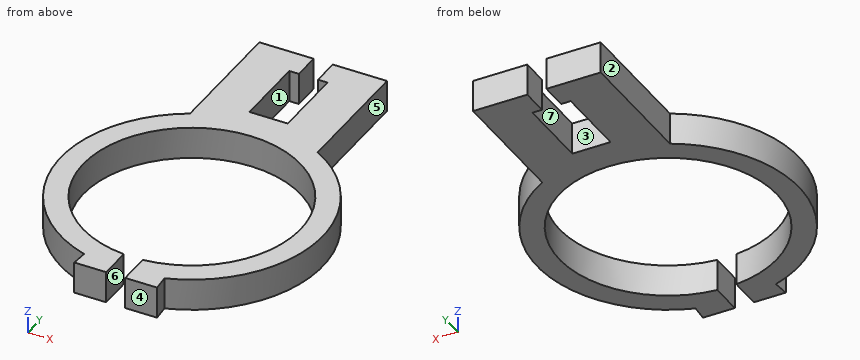
from build123d import *

# Parameters (mm, degrees)
SALIENTE_EXTRUIR1_DEPTH = 10


with BuildPart() as part:
    # Croquis1 → Saliente-Extruir1 (new body)
    with BuildSketch(Plane.XY):
        with BuildLine():
            Line((-20, 35.791060336), (-20, 75.791060336))
            Line((-20, 75.791060336), (-3, 75.791060336))
            Line((-3, 75.791060336), (-3, 67.291060336))
            Line((-3, 67.291060336), (-6, 67.291060336))
            Line((-6, 67.291060336), (-6, 44.291060336))
            Line((-6, 44.291060336), (-3, 44.291060336))
            Line((-3, 44.291060336), (3, 44.291060336))
            Line((3, 44.291060336), (6, 44.291060336))
            Line((6, 44.291060336), (6, 67.291060336))
            Line((6, 67.291060336), (3, 67.291060336))
            Line((3, 67.291060336), (3, 75.791060336))
            Line((3, 75.791060336), (20, 75.791060336))
            Line((20, 75.791060336), (20, 35.791060336))
            ThreePointArc((20, 35.791060336), (40.799890092, -4.04585819), (12.581284853, -39.02193321))
            Line((12.581284853, -39.02193321), (12.975031737, -44.006405438))
            Line((12.975031737, -44.006405438), (2.975031737, -44.006405438))
            Line((2.975031737, -44.006405438), (2.975031737, -40.891920793))
            Line((2.975031737, -40.891920793), (2.975031737, -33.869590877))
            ThreePointArc((2.975031737, -33.869590877), (0, 34), (-2.975031737, -33.869590877))
            Line((-2.975031737, -33.869590877), (-2.975031737, -40.891920793))
            Line((-2.975031737, -40.891920793), (-2.975031737, -44.006405438))
            Line((-2.975031737, -44.006405438), (-12.975031737, -44.006405438))
            Line((-12.975031737, -44.006405438), (-12.581284853, -39.02193321))
            ThreePointArc((-12.581284853, -39.02193321), (-40.799890092, -4.04585819), (-20, 35.791060336))
        make_face()
    extrude(amount=SALIENTE_EXTRUIR1_DEPTH)


solid = part.part
Geometry check sheet. Reference: the model listing, model coordinates, mm. Face numbers are marked on the shaded views. A direction names the side the tool comes from. Round coordinates to 2 decimals unless told otherwise and drop trailing zeros. Write each loop counter-clockwise with the first axis right and the second up, starting at its lowest first coordinate (ties: lowest second). Pieces come first, ordered by that corner, then holes.
Item 1: Mould release check, pull along Y, two halves, no side actions. Record for the marked faces 1, 2, 3 and 4: +Y half, -Y half, draft (parallel to the pull), parting line (faces both ways), or undercut.
Determined:
face 1: undercut
face 2: draft
face 3: undercut
face 4: -Y half
Item 2: Section check C-C (z = 7.5). Record the boundary of the cut face in (x, y), plus the area to 3 significant figures.
Determined:
outline: (-20, 35.79) arc R41 ccw to (-12.58, -39.02) - (-12.98, -44.01) - (-2.98, -44.01) - (-2.98, -33.87) arc R34 cw (long way) to (2.98, -33.87) - (2.98, -44.01) - (12.98, -44.01) - (12.58, -39.02) arc R41 ccw to (20, 35.79) - (20, 75.79) - (3, 75.79) - (3, 67.29) - (6, 67.29) - (6, 44.29) - (-6, 44.29) - (-6, 67.29) - (-3, 67.29) - (-3, 75.79) - (-20, 75.79) - close
area: 2,820 mm2
Item 3: Material ranges on line 1 along X through (y, z) = (0, 4.75); line 2 along X through (y, z) = (47, 5.25); line 3 along Y through (x, z) = (0, 7), recorded low to high.
Determined:
line 1: x = -41 to -34, 34 to 41
line 2: x = -20 to -6, 6 to 20
line 3: y = 34 to 44.29
Item 4: Access from +Z, -Z, +X, -X, +Y, -Y to the whole of each face (thin tool, end or side, straight path). Record for the marked faces 5, 6 and 7.
Determined:
face 5: +Z, -Z, +X, +Y
face 6: +Z, -Z, -Y
face 7: +Z, -Z
Item 5: Section check A-A (y = 64). Record the boundary of the cut face in (x, z), plus the area to 3 significant figures.
Determined:
outline: (-20, 0) - (-6, 0) - (-6, 10) - (-20, 10) - close; (6, 0) - (20, 0) - (20, 10) - (6, 10) - close
area: 280 mm2
Item 6: Go/stop test with flat-tipped pins: pin 1 Ø5 at (y, z) = (59.5, 7) entering from +X; pin 2 Ø3 at (y, z) = (54, 4) entering from -X; pin 3 Ø4 at (y, z) = (34, 2.5) entering from -X; pin 4 Ø8 at (x, y) = (23, 48.5) entering from -Z. Record where each tip stops, or that it passes through.
Determined:
pin 1: stops at x = 20
pin 2: stops at x = -20
pin 3: stops at x = -25.63
pin 4: stops at z = 0
Item 7: Section check D-D (x = 0). Record the boundary of the cut face in (y, z).
Determined:
outline: (34, 0) - (44.29, 0) - (44.29, 10) - (34, 10) - close
Item 8: Section check B-B (x = 15). Record the boundary of the cut face in (y, z).
Determined:
outline: (-38.16, 0) - (-30.51, 0) - (-30.51, 10) - (-38.16, 10) - close; (30.51, 0) - (75.79, 0) - (75.79, 10) - (30.51, 10) - close
